```python
from build123d import *

# Parameters (mm, degrees)
SKETCH2_R           = 12.5
BOSS_EXTRUDE1_DEPTH = 5
SKETCH4_R           = 12.5
BOSS_EXTRUDE2_DEPTH = 50


with BuildPart() as part:
    # Sketch2 → Revolve1 (revolve)
    with BuildSketch(Plane(origin=(0, 0, 0), x_dir=(1, 0, 0), z_dir=(0, 1, 0)), mode=Mode.PRIVATE) as revolve1_sk:
        with Locations((100, 0)):
            Circle(SKETCH2_R)
    revolve(revolve1_sk.sketch.rotate(Axis((0, 0, 0), (0, 0, 1)), 180), axis=Axis((0, 0, 0), (0, 0, 1)))

    # Sketch3 → Boss-Extrude1 (add, symmetric)
    with BuildSketch(Plane.XY):
        with BuildLine():
            Line((-73.52073385, -56.880972209), (-12.898955585, -21.880972209))
            ThreePointArc((-12.898955585, -21.880972209), (-21.997045256, -12.7), (-25.398955585, -0.230337114))
            Line((-25.398955585, -0.230337114), (-86.02073385, -35.230337114))
            Line((-86.02073385, -35.230337114), (-73.52073385, -56.880972209))
        make_face()
        with BuildLine():
            Line((-25.398955585, -0.230337114), (-12.898955585, -21.880972209))
            ThreePointArc((-12.898955585, -21.880972209), (0, -25.4), (12.898955585, -21.880972209))
            Line((12.898955585, -21.880972209), (25.398955585, -0.230337114))
            ThreePointArc((25.398955585, -0.230337114), (25.399738895, -0.115169741), (25.4, 0))
            ThreePointArc((25.4, 0), (21.939234262, 12.799609369), (12.5, 22.111309324))
            Line((12.5, 22.111309324), (-12.5, 22.111309324))
            ThreePointArc((-12.5, 22.111309324), (-21.997045256, 12.7), (-25.398955585, -0.230337114))
        make_face()
        with BuildLine():
            ThreePointArc((-25.398955585, -0.230337114), (-21.997045256, -12.7), (-12.898955585, -21.880972209))
            Line((-12.898955585, -21.880972209), (-25.398955585, -0.230337114))
        make_face()
        with BuildLine():
            ThreePointArc((12.5, 22.111309324), (0, 25.4), (-12.5, 22.111309324))
            Line((-12.5, 22.111309324), (12.5, 22.111309324))
        make_face()
        with BuildLine():
            Line((-12.5, 92.111309324), (-12.5, 22.111309324))
            ThreePointArc((-12.5, 22.111309324), (0, 25.4), (12.5, 22.111309324))
            Line((12.5, 22.111309324), (12.5, 92.111309324))
            Line((12.5, 92.111309324), (-12.5, 92.111309324))
        make_face()
        with BuildLine():
            Line((25.398955585, -0.230337114), (12.898955585, -21.880972209))
            ThreePointArc((12.898955585, -21.880972209), (21.997045256, -12.7), (25.398955585, -0.230337114))
        make_face()
        with BuildLine():
            ThreePointArc((25.398955585, -0.230337114), (21.997045256, -12.7), (12.898955585, -21.880972209))
            Line((12.898955585, -21.880972209), (73.52073385, -56.880972209))
            Line((73.52073385, -56.880972209), (86.02073385, -35.230337114))
            Line((86.02073385, -35.230337114), (25.398955585, -0.230337114))
        make_face()
    extrude(amount=BOSS_EXTRUDE1_DEPTH, both=True)

    # Sketch4 → Boss-Extrude2 (add)
    with BuildSketch(Plane(origin=(0, 0, -5), x_dir=(-1, 0, 0), z_dir=(0, 0, -1))):
        with Locations(Location((0, 0, 0), (0, 0, 180))):
            Circle(SKETCH4_R)
    extrude(amount=BOSS_EXTRUDE2_DEPTH)


solid = part.part
```
Here's how the part is built. I have some questions about the finished solid (model axes, mm). A direction names the side the tool comes from. Coordinates: 2 decimals unless noted, no trailing zeros. Write each loop counter-clockwise with the first axis right and the second up, starting at its lowest first coordinate (ties: lowest second). Pieces come first, ordered by that corner, then holes. Notation, with made-up numbers: (-36.5, 45) -> (18.5, 45) arc R33 cw to (18.5, 75) -> close; hole circle Ø7 at (57, -2.75). An arc over 180 degrees is marked (long way). Use a Markdown table: item, result. Add a question column.
(1) If we section it at A-A, the plane z = -37: Write out the boundary of the cut face in (x, y).
(2) Please list where these lines run through material, in increasing order: line 1 (Y direction, x = -8, z = -8); line 2 (Z direction, x = -98, y = 12); line 3 (Z direction, x = 23.5, y = -15.5).
(3) We'd pull the mould along X, two halves only. Please class faces 4 (the flat face through (-12.5, 55, 0)), 5 (the flat face through (54.178, -16.846, 0.07)), 6 (the flat face through (0, 0, -55)): +X half, -X half, draft (parallel to the pull), parting line (faces both ways), or undercut.
(4) For faces 1 (the flat face through (0, -4, 5)), 2 (the cylindrical face through (22.03, 12.64, 0.07)), 3 (the cylindrical face through (11.923, -3.755, -29.65)), which set-ups out of +Z, -Z, +X, -X, +Y, -Y let a thin tool reach every point of the face, with its end or its side?
(5) If we section it at B-B, the plane y = 82.5: State how many separate pieces and enclosed holes the cut face has, and give its area (3 significant figures).
(6) I'm going to push flat-ended pins straight in: P1, Ø2, axis at x = -84, y = -50.5, coming from the -Z side; P2, Ø6, axis at y = -82, z = -1, coming from the +X side; P3, Ø10, axis at x = 14.5, y = 46, coming from the +Z side. Where does each tip first touch, or does it pass through?
Outcome:
| question | item | result |
|---|---|---|
| 1 | outline | circle Ø25 at (0, 0) |
| 2 | line 1 | y = -109.31 to -90.04, -9.6 to 9.6, 90.04 to 109.31 |
| 2 | line 2 | z = -12.44 to 12.44 |
| 2 | line 3 | z = -5 to 5 |
| 3 | face 4 | undercut |
| 3 | face 5 | undercut |
| 3 | face 6 | draft |
| 4 | face 1 | +Z |
| 4 | face 2 | +Z, -Z |
| 4 | face 3 | -Z |
| 5 | separate pieces | 3 |
| 5 | enclosed holes | 0 |
| 5 | area | 2,070 mm^2 |
| 6 | P1 | stops at z = -12.46 |
| 6 | P2 | stops at x = 80.05 |
| 6 | P3 | stops at z = 5 |
